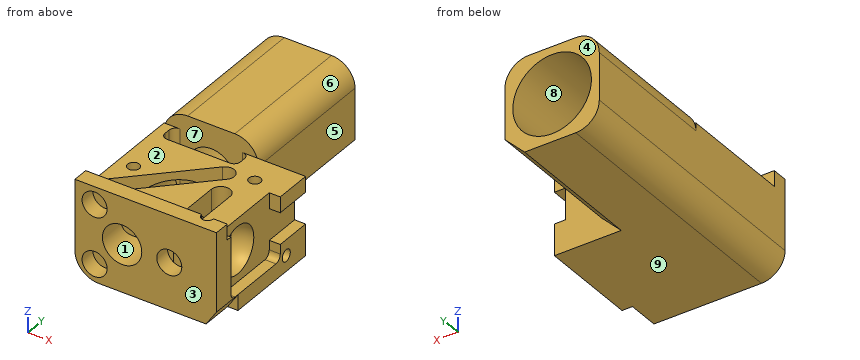
```python
from build123d import *

# Parameters (mm, degrees)
SKETCH1_W                   = 9
SKETCH1_H                   = 6
MAIN_BODY_EXT_DEPTH         = 8.3
EMISSION_PATH_EXT_DEPTH     = 9
SKETCH3_R                   = 1.25
EMISSION_AND_GRIN_CUT_DEPTH = 19.125672401
SKETCH4_R                   = 1
DRUM_LENS_CUT_DEPTH         = 7
SKETCH5_W                   = 9
SKETCH5_H                   = 7.3
FILTERSET_CUT1_DEPTH        = 1
FILTERSET_CUT2_DEPTH        = 4
SKETCH10_R                  = 2.5
EMISSION_LENS_CUT_DEPTH     = 8.5
SKETCH15_R                  = 0.795
MAGNETS_CUT_DEPTH           = 1
SCREW_HOLES_CUT_DEPTH       = 19.561788707
SCREW_HOLES_CUT_DEPTH_BACK  = 3
SKETCH18_R                  = 0.375
EXTERNAL_FILLET_1_R         = 1.5
CUT_EXTRUDE8_DEPTH          = 12.545128843
CUT_EXTRUDE8_DEPTH_BACK     = 4
SKETCH28_R                  = 1.5
CUT_EXTRUDE9_DEPTH          = 2
CUT_EXTRUDE10_DEPTH         = 0.7
SKETCH29_R                  = 0.375
CUT_EXTRUDE11_DEPTH         = 2.5
SKETCH32_W                  = 2
SKETCH32_H                  = 2.36
CUT_EXTRUDE14_DEPTH         = 0.7
CUT_EXTRUDE16_DEPTH         = 9


with BuildPart() as part:
    # Sketch1 → Main Body Ext (new body)
    with BuildSketch(Plane(origin=(0, 0, 0), x_dir=(1, 0, 0), z_dir=(0, 1, 0))):
        Rectangle(SKETCH1_W, SKETCH1_H)
    extrude(amount=MAIN_BODY_EXT_DEPTH)

    # Sketch8 → Emission Path Ext (add)
    with BuildSketch(Plane(origin=(0, 8.3, 0), x_dir=(1, 0, 0), z_dir=(0, 1, 0))):
        Polygon((0.25, 3), (1.5, 1.75), (1.5, -3), (-4.5, -3), (-4.5, 3), align=None)
    extrude(amount=EMISSION_PATH_EXT_DEPTH)

    # Sketch3 → Emission and Grin Cut (cut, through all)
    with BuildSketch(Plane.XZ):
        with Locations(Location((-1.5, 0, 0), (0, 0, 270))):
            Circle(SKETCH3_R)
    extrude(amount=-EMISSION_AND_GRIN_CUT_DEPTH, mode=Mode.SUBTRACT)

    # Sketch4 → Drum Lens Cut (cut)
    with BuildSketch(Plane(origin=(4.5, 0, 0), x_dir=(0, 0, -1), z_dir=(1, 0, 0))):
        with Locations((0, 3)):
            Circle(SKETCH4_R)
    extrude(amount=-DRUM_LENS_CUT_DEPTH, mode=Mode.SUBTRACT)

    # Sketch5 → FilterSet Cut1 (cut)
    with BuildSketch(Plane.XY.offset(3)):
        with Locations((0, 4.65)):
            Rectangle(SKETCH5_W, SKETCH5_H)
    extrude(amount=-FILTERSET_CUT1_DEPTH, mode=Mode.SUBTRACT)

    # Sketch6 → FilterSet Cut2 (cut)
    with BuildSketch(Plane.XY.offset(2)):
        with BuildLine():
            Line((2.3, 4.5), (2.3, 1.8))
            ThreePointArc((2.3, 1.8), (2.7, 1.4), (2.3, 1))
            Line((2.3, 1), (1.1, 1))
            ThreePointArc((1.1, 1), (0.7, 1.4), (1.1, 1.8))
            Line((1.1, 1.8), (1.1, 4.5))
            ThreePointArc((1.1, 4.5), (1.7, 5.1), (2.3, 4.5))
        make_face()
        with BuildLine():
            Line((-3.9, 7.9), (-3.9, 7.5))
            ThreePointArc((-3.9, 7.5), (-3.782842712, 7.217157288), (-3.5, 7.1))
            Line((-3.5, 7.1), (0.5, 7.1))
            ThreePointArc((0.5, 7.1), (0.782842712, 7.217157288), (0.9, 7.5))
            Line((0.9, 7.5), (0.9, 7.9))
            ThreePointArc((0.9, 7.9), (0.782842712, 8.182842712), (0.5, 8.3))
            Line((0.5, 8.3), (-3.5, 8.3))
            ThreePointArc((-3.5, 8.3), (-3.782842712, 8.182842712), (-3.9, 7.9))
        make_face()
        with BuildLine():
            Line((0.39411255, 6.591168825), (-3.848528137, 2.348528137))
            ThreePointArc((-3.848528137, 2.348528137), (-3.848528137, 1.5), (-3, 1.5))
            Line((-3, 1.5), (1.242640687, 5.742640687))
            ThreePointArc((1.242640687, 5.742640687), (1.242640687, 6.591168825), (0.39411255, 6.591168825))
        make_face()
    extrude(amount=-FILTERSET_CUT2_DEPTH, mode=Mode.SUBTRACT)

    # Sketch10 → Emission Lens Cut (cut)
    with BuildSketch(Plane(origin=(0, 17.3, 0), x_dir=(1, 0, 0), z_dir=(0, 1, 0))):
        with Locations(Location((-1.5, 0, 0), (0, 0, 270))):
            Circle(SKETCH10_R)
    extrude(amount=-EMISSION_LENS_CUT_DEPTH, mode=Mode.SUBTRACT)

    # Sketch15 → Magnets Cut (cut)
    with BuildSketch(Plane.XZ):
        with Locations(Location((-3.25, -1.875, 0), (0, 0, 270))):
            Circle(SKETCH15_R)
        with Locations(Location((-3.25, 1.875, 0), (0, 0, 270))):
            Circle(SKETCH15_R)
        with Locations(Location((1.5, 0, 0), (0, 0, 270))):
            Circle(SKETCH15_R)
    extrude(amount=-MAGNETS_CUT_DEPTH, mode=Mode.SUBTRACT)

    # Sketch18 → Screw Holes Cut (cut, two sides: drawn at the far end of the back side and taken through both)
    with BuildSketch(Plane.XY.offset(2).offset(-SCREW_HOLES_CUT_DEPTH_BACK)):
        with Locations(Location((-3.5, 4, 0), (0, 0, 180))):
            Circle(SKETCH18_R)
        with Locations(Location((2.5, 6.5, 0), (0, 0, 180))):
            Circle(SKETCH18_R)
        with Locations((3.25, 1)):
            Circle(SKETCH18_R)
    extrude(amount=SCREW_HOLES_CUT_DEPTH + SCREW_HOLES_CUT_DEPTH_BACK, mode=Mode.SUBTRACT)

    # External Fillet 1
    # the kernel refuses this fillet: 1.5 mm, written as the material it takes off along each edge
    with BuildSketch(Plane(origin=(-4.5, -3.75, -3), x_dir=(1, 0, 0), z_dir=(0, 1, 0))) as external_fillet_1_piece_1:
        with BuildLine():
            CenterArc((EXTERNAL_FILLET_1_R, -EXTERNAL_FILLET_1_R), EXTERNAL_FILLET_1_R, 90, 90)
            Line((0, -EXTERNAL_FILLET_1_R), (0, 0))
            Line((0, 0), (EXTERNAL_FILLET_1_R, 0))
        make_face()
    extrude(amount=24.8, mode=Mode.SUBTRACT)
    with BuildSketch(Plane(origin=(1.5, 8.3, 3), x_dir=(0, 0, -1), z_dir=(0, 1, 0))) as external_fillet_1_piece_2:
        with BuildLine():
            CenterArc((EXTERNAL_FILLET_1_R, EXTERNAL_FILLET_1_R), EXTERNAL_FILLET_1_R, 180, 90)
            Line((0, EXTERNAL_FILLET_1_R), (0, 0))
            Line((0, 0), (EXTERNAL_FILLET_1_R, 0))
        make_face()
    extrude(amount=12.75, mode=Mode.SUBTRACT)

    # Sketch28 → Cut-Extrude8 (cut, two sides: drawn at the far end of the back side and taken through both)
    with BuildSketch(Plane(origin=(0, 7.1, 0), x_dir=(1, 0, 0), z_dir=(0, 1, 0)).offset(-CUT_EXTRUDE8_DEPTH_BACK)):
        with Locations(Location((-1.5, 0, 0), (0, 0, 180))):
            Circle(SKETCH28_R)
    extrude(amount=CUT_EXTRUDE8_DEPTH + CUT_EXTRUDE8_DEPTH_BACK, mode=Mode.SUBTRACT)

    # Sketch14 → Cut-Extrude9 (cut)
    with BuildSketch(Plane.XZ):
        Polygon((4.5, -3), (4.5, -2.006698359), (3.837798906, -3), align=None)
    extrude(amount=-CUT_EXTRUDE9_DEPTH, mode=Mode.SUBTRACT)

    # Sketch12 → Cut-Extrude10 (cut)
    with BuildSketch(Plane(origin=(4.5, 0, 0), x_dir=(0, 0, -1), z_dir=(1, 0, 0))):
        with BuildLine():
            Line((1.6, 5.94), (-1.6, 5.94))
            Line((-1.6, 5.94), (-2, 5.94))
            Line((-2, 5.94), (-2, 1.33))
            Line((-2, 1.33), (1.6, 1.33))
            ThreePointArc((1.6, 1.33), (1.882842712, 1.447157288), (2, 1.73))
            Line((2, 1.73), (2, 5.54))
            ThreePointArc((2, 5.54), (1.882842712, 5.822842712), (1.6, 5.94))
        make_face()
    extrude(amount=-CUT_EXTRUDE10_DEPTH, mode=Mode.SUBTRACT)

    # Sketch29 → Cut-Extrude11 (cut)
    with BuildSketch(Plane(origin=(4.5, 0, 0), x_dir=(0, 0, -1), z_dir=(1, 0, 0))):
        with Locations((2, 6.5)):
            Circle(SKETCH29_R)
    extrude(amount=-CUT_EXTRUDE11_DEPTH, mode=Mode.SUBTRACT)

    # Sketch32 → Cut-Extrude14 (cut)
    with BuildSketch(Plane(origin=(4.5, 0, 0), x_dir=(0, 0, -1), z_dir=(1, 0, 0))):
        with Locations((0, 7.12)):
            Rectangle(SKETCH32_W, SKETCH32_H)
    extrude(amount=-CUT_EXTRUDE14_DEPTH, mode=Mode.SUBTRACT)

    # Sketch33 → Cut-Revolve1 (revolve, cut)
    with BuildSketch(Plane.XY, mode=Mode.PRIVATE) as cut_revolve1_sk:
        with BuildLine():
            Line((3.8, 3), (2.3, 3))
            ThreePointArc((2.3, 3), (2.739339828, 4.060660172), (3.8, 4.5))
            Line((3.8, 4.5), (3.8, 3))
        make_face()
    revolve(cut_revolve1_sk.sketch.rotate(Axis((3.8, 3, 0), (-1, 0, 0)), 90), axis=Axis((3.8, 3, 0), (-1, 0, 0)), mode=Mode.SUBTRACT)

    # Sketch36 → Cut-Extrude16 (cut)
    with BuildSketch(Plane(origin=(0, 17.3, 0), x_dir=(1, 0, 0), z_dir=(0, 1, 0))):
        with BuildLine():
            Line((-4.5, -1.5), (-4.5, -3))
            Line((-4.5, -3), (-3, -3))
            ThreePointArc((-3, -3), (-4.060660172, -2.560660172), (-4.5, -1.5))
        make_face()
    extrude(amount=-CUT_EXTRUDE16_DEPTH, mode=Mode.SUBTRACT)


solid = part.part
```
Work out the finished part from the listing and answer in its coordinate system (mm). Face numbers are marked on the shaded views. A direction names the side the tool comes from. Give positions to 0.01 mm unless a question says otherwise; leave off trailing zeros. Order: outer loops, then holes, each group sorted by start corner. A loop starts at its lowest first (then second) coordinate and runs counter-clockwise, first axis right, second up. Notation, with made-up numbers: M 38,9 L 97,9 A31 cw 97,35 Z; hole C 18.25,67 d2. An arc over 180 degrees is marked long. Return JSON: item names as keys, results as strings.
1) Section C-C, the plane x = -1.75 is taken. Give the number of separate pieces and of enclosed holes in the cut face, plus the area to 3 significant figures.
Resolved:
{"separate pieces": "4", "enclosed holes": "0", "area": "26.6 mm^2"}
2) Section D-D, the plane y = 4.75 is taken. Write down the section's boundary in (x, z), plus the area to 3 significant figures.
Resolved:
{"outline": "M -4.5,-1.5 A1.5 ccw -3,-3 L 4.5,-3 L 4.5,-2 L 3.8,-2 L 3.8,2 L 2.25,2 L 2.25,-2 L 1.15,-2 L 1.15,2 L 0.25,2 L 0.25,-2 L -1.45,-2 L -1.45,-1.5 A1.5 cw long -1.45,1.5 L -1.45,2 L -4.5,2 Z", "area": "26.9 mm^2"}
3) A tool of negligible diameter and unlimited length cuts with its end or side. For the marked faces 5, 6, 7, 8 and 9, from which of +Z, -Z, +X, -X, +Y, -Y can it reach the whole face along a straight path? Write none if from no direction.
Resolved:
{"face 5": "+Z, -Z, +X, +Y", "face 6": "+Z, +X, +Y", "face 7": "+Z", "face 8": "+Y", "face 9": "-Z, +X, -X, +Y, -Y"}
4) Section A-A, the plane x = 1.75 is taken. Write down the section's boundary in (y, z).
Resolved:
{"outline": "M 0,-3 L 8.3,-3 L 8.3,2 L 5.1,2 L 5.1,-2 L 1,-2 L 1,-0.75 L 0,-0.75 Z; M 0,0.75 L 1,0.75 L 1,3 L 0,3 Z"}
5) Each of these flat-tipped pins is pushed along its axis until it touches: pin 1 (2 mm diameter, centred on x = 2, y = 6, fed in from +Z); pin 2 (2.5 mm diameter, centred on x = -1, z = 1, fed in from +Y). Where does it stop, or does it pass through?
Resolved:
{"pin 1": "z = 2", "pin 2": "y = 8.8"}
6) Section B-B, the plane y = 13.5 is taken. Write down the section's boundary in (x, z).
Resolved:
{"outline": "M -4.5,-1.5 A1.5 ccw -3,-3 L 0.25,-3 L 1.5,-1.75 L 1.5,1.5 A1.5 ccw 0,3 L -3,3 A1.5 ccw -4.5,1.5 Z; hole C -1.5,0 d5"}
7) Straight lines are drawn through the part: line 1 along Y through (x, z) = (-3, 0.55); line 2 along X through (y, z) = (0.95, 0) (3 decimals); line 3 along Y through (x, z) = (4, 1.2). For each, find the intervals that lie inside material, in ascending order. Write a range as [from, to].
Resolved:
{"line 1": "[0, 1.5], [3.2, 7.1], [8.3, 8.8]", "line 2": "[-4.5, -2.75], [-0.25, 0.705], [2.295, 2.878], [3.622, 4.5]", "line 3": "[0, 1.33], [5.94, 8.3]"}
8) For a pull along Y with two mould halves and no side action, classify the marked faces 1, 2, 3 and 4 as +Y half, -Y half, draft (parallel to the pull), parting line (faces both ways), or undercut.
Resolved:
{"face 1": "draft", "face 2": "undercut", "face 3": "-Y half", "face 4": "+Y half"}
